Design review of the part built by this model. Coordinates are the model's own, in mm. A direction names the side the tool comes from. Coordinates: 2 decimals unless noted, no trailing zeros. Order: outer loops, then holes, each group sorted by start corner. A loop starts at its lowest first (then second) coordinate and runs counter-clockwise, first axis right, second up. Notation, with made-up numbers: M -19.5,46.5 L 17.5,46.5 A16 cw 17.5,66.5 Z; hole C -3.75,21.5 d10. An arc over 180 degrees is marked long. Answer in a Markdown table with one row per item.
from build123d import *

# Parameters (mm, degrees)
F0_R     = 1.905
F1_DEPTH = 19.05
F2_R     = 2.413
F3_DEPTH = 2.413
F5_DEPTH = 2.7686


with BuildPart() as f1:
    # F0 (on Front) → F1 (new body)
    with BuildSketch(Plane.XZ):
        Circle(F0_R)
    extrude(amount=F1_DEPTH)

    # F2 (on face) → F3 (join)
    with BuildSketch(Plane.XZ.offset(19.05)):
        Circle(F2_R)
    extrude(amount=F3_DEPTH)

    # F4 (on face) → F5 (cut)
    with BuildSketch(Plane.XZ.offset(21.463)):
        Polygon((-0.00353, 1.389058), (-1.204725, 0.691472), (-1.201194, -0.697586), (0.00353, -1.389058), (1.204725, -0.691472), (1.201194, 0.697586), align=None)
    extrude(amount=-F5_DEPTH, mode=Mode.SUBTRACT)


solid = f1.part
(1) Insertion check: pin 1 Ø1 at (x, y) = (0.5, -6.5) entering from +Z (3 decimals); pin 2 Ø2 at (x, y) = (1, -2.5) entering from -Z (3 decimals). Each pin has a flat end and moves straight along its axis. Give the tip position at first contact, or say it passes through.
Return value:
| item | result |
|---|---|
| pin 1 | stops at z = 1.905 |
| pin 2 | stops at z = -1.905 |
(2) Add section B-B, the plane z = -0.9. Give the boundary of the cut face in (x, y).
Return value:
| item | result |
|---|---|
| outline | M -2.24,-21.46 L -0.85,-21.46 L -0.85,-18.69 L 0.85,-18.69 L 0.85,-21.46 L 2.24,-21.46 L 2.24,-19.05 L 1.68,-19.05 L 1.68,0 L -1.68,0 L -1.68,-19.05 L -2.24,-19.05 Z |
(3) Add section C-C, the plane y = -14. Give the boundary of the cut face in (x, z) (3 decimals), and give its area (3 significant figures).
Return value:
| item | result |
|---|---|
| outline | C 0,0 d3.81 |
| area | 11.4 mm2 |
(4) For line 1 along Y through (x, z) = (-0.35, 2.2); line 2 along Y through (x, z) = (0, -0.85); line 3 along Z through (x, y) = (0.7, -19), list the stretches that pass through material, from the lowest coordinate up. Write a range as from..to.
Return value:
| item | result |
|---|---|
| line 1 | y = -21.46..-19.05 |
| line 2 | y = -18.69..0 |
| line 3 | z = -1.77..-0.98, 0.99..1.77 |
(5) For faces 4 (the flat face through (2, -19.05, 1)), 5 (the flat face through (0.596, -20.098, -1.045)), 6 (the flat face through (1, -21.463, 1)), list the 3-axis set-ups (+Z, -Z, +X, -X, +Y, -Y) from which the entire face can be reached by the end or side of a thin tool; tool diameter is ignored.
Return value:
| item | result |
|---|---|
| face 4 | +Y |
| face 5 | -Y |
| face 6 | +Z, -Z, +X, -X, -Y |
(6) Add section D-D, the plane z = 0. Give the boundary of the cut face in (x, y) (3 decimals), and give its area (3 significant figures).
Return value:
| item | result |
|---|---|
| outline | M -2.413,-21.463 L -1.203,-21.463 L -1.203,-18.694 L 1.203,-18.694 L 1.203,-21.463 L 2.413,-21.463 L 2.413,-19.05 L 1.905,-19.05 L 1.905,0 L -1.905,0 L -1.905,-19.05 L -2.413,-19.05 Z |
| area | 77.6 mm2 |
(7) Draft analysis for pull direction X (two halves, no side actions). For faces 1 (the cylindrical face through (-0.41, -9.39, -1.86)), 2 (the flat face through (-0.607, -20.098, -1.038)), 3 (the flat face through (0, 0, 0)), state which applies: pulls with the +X half, pulls with the -X half, needs draft (parallel to the pull), parting line crosses it, or undercut.
Return value:
| item | result |
|---|---|
| face 1 | parting line crosses it |
| face 2 | undercut |
| face 3 | needs draft |
(8) Add section A-A, the plane x = -1.4. Give the boundary of the cut face in (y, z), and give its area (3 significant figures).
Return value:
| item | result |
|---|---|
| outline | M -21.46,-1.97 L -19.05,-1.97 L -19.05,-1.29 L 0,-1.29 L 0,1.29 L -19.05,1.29 L -19.05,1.97 L -21.46,1.97 Z |
| area | 58.7 mm2 |
